from build123d import *

# Parameters (mm, degrees)
SKETCH1_R           = 4.75
BOSS_EXTRUDE1_DEPTH = 70
CUT_EXTRUDE1_DEPTH  = 10
CUT_EXTRUDE2_DEPTH  = 71.39132475
CUT_EXTRUDE3_REACH  = 72.322
SKETCH5_W           = 1
SKETCH5_H           = 70
CUT_EXTRUDE4_DEPTH  = 1.5
SKETCH6_R           = 1
BOSS_EXTRUDE2_DEPTH = 5


with BuildPart() as part:
    # Sketch1 → Boss-Extrude1 (new body)
    with BuildSketch(Plane.XY):
        Circle(SKETCH1_R)
    extrude(amount=BOSS_EXTRUDE1_DEPTH)

    # Sketch2 → Cut-Extrude1 (cut)
    with BuildSketch(Plane(origin=(0, 0, 0), x_dir=(-1, 0, 0), z_dir=(0, 0, -1))):
        with BuildLine():
            Line((-0.94, 1.535057002), (-0.94, -1.535057002))
            ThreePointArc((-0.94, -1.535057002), (1.8, 0), (-0.94, 1.535057002))
        make_face()
    extrude(amount=-CUT_EXTRUDE1_DEPTH, mode=Mode.SUBTRACT)

    # Sketch3 → Cut-Extrude2 (cut, through all)
    with BuildSketch(Plane.ZY.offset(-0.94)):
        Polygon((3.230708553, 0.754115238), (1.962271323, 1.44288249), (0.73156277, 0.688767252), (0.769291447, -0.754115238), (2.037728677, -1.44288249), (3.26843723, -0.688767252), align=None)
    extrude(amount=-CUT_EXTRUDE2_DEPTH, mode=Mode.SUBTRACT)

    # Sketch4 → Cut-Extrude3 (cut, up to next)
    with BuildSketch(Plane(origin=(0, 0, 0), x_dir=(-1, 0, 0), z_dir=(0, 0, -1)), mode=Mode.PRIVATE) as cut_extrude3_sk1:
        with BuildLine():
            Line((-3.682729966, 3), (3.682729966, 3))
            ThreePointArc((3.682729966, 3), (0, 4.75), (-3.682729966, 3))
        make_face()
    cut_extrude3_tool1 = extrude(cut_extrude3_sk1.sketch, amount=-CUT_EXTRUDE3_REACH, mode=Mode.PRIVATE) & part.part
    # Sketch4 → Cut-Extrude3 (cut, up to next)
    with BuildSketch(Plane(origin=(0, 0, 0), x_dir=(-1, 0, 0), z_dir=(0, 0, -1)), mode=Mode.PRIVATE) as cut_extrude3_sk2:
        with BuildLine():
            Line((-3.682729966, -3), (3.682729966, -3))
            ThreePointArc((3.682729966, -3), (0, -4.75), (-3.682729966, -3))
        make_face()
    cut_extrude3_tool2 = extrude(cut_extrude3_sk2.sketch, amount=-CUT_EXTRUDE3_REACH, mode=Mode.PRIVATE) & part.part
    add(cut_extrude3_tool1.solids().sort_by_distance((0, 3.712383, 0))[0], mode=Mode.SUBTRACT)
    add(cut_extrude3_tool2.solids().sort_by_distance((0, -3.712383, 0))[0], mode=Mode.SUBTRACT)

    # Sketch5 → Cut-Extrude4 (cut)
    with BuildSketch(Plane(origin=(0, 3, 0), x_dir=(1, 0, 0), z_dir=(0, 1, 0))):
        with Locations((0, -35)):
            Rectangle(SKETCH5_W, SKETCH5_H)
    cut_extrude4 = extrude(amount=-CUT_EXTRUDE4_DEPTH, mode=Mode.SUBTRACT)

    # Mirror1: Cut-Extrude4 across plane
    add(cut_extrude4.mirror(Plane.ZX), mode=Mode.SUBTRACT)

    # Sketch6 → Boss-Extrude2 (add)
    with BuildSketch(Plane.XY.offset(70)):
        Circle(SKETCH6_R)
    extrude(amount=BOSS_EXTRUDE2_DEPTH)


solid = part.part
Can you work these out from the model? Positions are in its coordinate system, mm. A direction names the side the tool comes from. Give positions to 0.01 mm unless a question says otherwise; leave off trailing zeros. Write each loop counter-clockwise with the first axis right and the second up, starting at its lowest first coordinate (ties: lowest second). Pieces come first, ordered by that corner, then holes. Notation, with made-up numbers: M 43.5,-13.75 L 56.5,-13.75 A17 cw 56.5,-3.75 Z; hole C 19.5,55 d3. An arc over 180 degrees is marked long. Answer in a Markdown table with one row per item. Add a question column.
Item 1: Imagine slicing it at A-A, the plane z = 59.5. Write out the boundary of the cut face in (x, y).
Item 2: On a 3-axis mill with a long thin cutter (end or side, diameter ignored), from which of +Z, -Z, +X, -X, +Y, -Y can I reach the whole of each face in a straight line? I mean faces 4 (the flat face through (2.8, 1.1, 1.4)), 5 (the cylindrical face through (0, -1, 72)), 6 (the flat face through (2, -3, 35)), 7 (the cylindrical face through (-1.8, 0, 4.9)), 8 (the flat face through (0.5, -2, 35)). Say none if no direction works.
Item 3: Imagine slicing it at C-C, the plane x = -2.75. Write out the boundary of the cut face in (y, z), plus the area to 3 significant figures.
Item 4: We'd pull the mould along Z, two halves only. Please class faces 1 (the flat face through (1, -1, 70)), 2 (the flat face through (2.79, -1.09, 1.39)), 3 (the flat face through (3, 0, 0)): released by +Z, released by -Z, zero draft, split by the parting line, or undercut.
Item 5: For pin 1 Ø1.6 at (y, z) = (2.5, 19.5) entering from +X; pin 2 Ø2 at (y, z) = (-1.5, 61.5) entering from +X; pin 3 Ø1.2 at (y, z) = (-2, 43) entering from +X, each with a flat end and sliding along its axis, tell me the tip position at first contact or that it passes through.
Item 6: Please list where these lines run through material, in increasing order: L1, parallel to X at y = 2.15, z = 42.5; L2, parallel to Z at x = -1.5, y = -2.4; L3, parallel to X at y = -1.8, z = 38.
Item 7: Imagine slicing it at B-B, the plane y = 0. Write out the boundary of the cut face in (x, z), plus the area to 3 significant figures.
Evaluation:
| question | item | result |
|---|---|---|
| 1 | outline | M -3.68,-3 L -0.5,-3 L -0.5,-1.5 L 0.5,-1.5 L 0.5,-3 L 3.68,-3 A4.75 ccw 3.68,3 L 0.5,3 L 0.5,1.5 L -0.5,1.5 L -0.5,3 L -3.68,3 A4.75 ccw Z |
| 2 | face 4 | +X |
| 2 | face 5 | +Z |
| 2 | face 6 | +Z, -Z, +X, -X, -Y |
| 2 | face 7 | -Z |
| 2 | face 8 | +Z, -Z, -Y |
| 3 | outline | M -3,0 L 3,0 L 3,70 L -3,70 Z |
| 3 | area | 420 mm² |
| 4 | face 1 | released by +Z |
| 4 | face 2 | undercut |
| 4 | face 3 | released by -Z |
| 5 | pin 1 | stops at x = 4.44 |
| 5 | pin 2 | stops at x = 4.72 |
| 5 | pin 3 | stops at x = 4.54 |
| 6 | L1 | x = -4.24 to -0.5, 0.5 to 4.24 |
| 6 | L2 | z = 0 to 70 |
| 6 | L3 | x = -4.4 to -0.5, 0.5 to 4.4 |
| 7 | outline | M -4.75,0 L -1.8,0 L -1.8,10 L 0.94,10 L 0.94,3.25 L 4.75,3.25 L 4.75,70 L 1,70 L 1,75 L -1,75 L -1,70 L -4.75,70 Z; M 0.94,0 L 4.75,0 L 4.75,0.75 L 0.94,0.75 Z |
| 7 | area | 638 mm² |
